Design review of the part built by this model. Coordinates are the model's own, in mm. A direction names the side the tool comes from. Give positions to 0.01 mm unless a question says otherwise; leave off trailing zeros. Loops run counter-clockwise (first coordinate to the right, second up) from the corner with the lowest first, then second, coordinate; pieces in that order, holes last.
Autodesk Inventor part; units mm, degrees
ref_plane "YZ Plane" through (0, 0, 0) normal (1, 0, 0) x (0, 1, 0)
ref_plane "XZ Plane" through (0, 0, 0) normal (0, 1, 0) x (-1, 0, 0)
ref_plane "XY Plane" through (0, 0, 0) normal (0, 0, 1) x (1, 0, 0)
sketch "スケッチ2" plane through (0, 0, 0) normal (0, 1, 0) x (-1, 0, 0)
  line L0 (-32.5, -11.25) -> (32.5, -11.25)
  line L1 (32.5, -11.25) -> (32.5, 11.25)
  line L2 (32.5, 11.25) -> (-32.5, 11.25)
  line L3 (-32.5, 11.25) -> (-32.5, -11.25)
  line L4 (-32.5, -11.25) -> (32.5, 11.25) construction
  line L5 (32.5, -11.25) -> (-32.5, 11.25) construction
  line L6 (-30, -8.75) -> (30, -8.75)
  line L7 (30, -8.75) -> (30, 8.75)
  line L8 (30, 8.75) -> (-30, 8.75)
  line L9 (-30, 8.75) -> (-30, -8.75)
  line L10 (-30, -8.75) -> (30, 8.75) construction
  line L11 (30, -8.75) -> (-30, 8.75) construction
  circle A0 centre (30, 8.75) radius 2.5
  circle A1 centre (30, -8.75) radius 2.5
  circle A2 centre (-30, 8.75) radius 2.5
  circle A3 centre (-30, -8.75) radius 2.5
  line L12 (-115, -18.25) -> (115, -18.25)
  line L13 (115, -18.25) -> (115, 18.25)
  line L14 (115, 18.25) -> (-115, 18.25)
  line L15 (-115, 18.25) -> (-115, -18.25)
  line L16 (-115, -18.25) -> (115, 18.25) construction
  line L17 (115, -18.25) -> (-115, 18.25) construction
  line L18 (-95, -18.25) -> (95, -18.25)
  line L19 (95, -18.25) -> (95, 18.25)
  line L20 (95, 18.25) -> (-95, 18.25)
  line L21 (-95, 18.25) -> (-95, -18.25)
  line L22 (-95, -18.25) -> (95, 18.25) construction
  line L23 (95, -18.25) -> (-95, 18.25) construction
  point P0 (0, 0)
  dimension "d10" = 65
  dimension "d11" = 22.5
  dimension "d12" = 60
  dimension "d13" = 17.5
  dimension "d14" = 230
  dimension "d15" = 36.5
  dimension "d16" = 190
sketch "スケッチ4" plane through (0, 0, 0) normal (1, 0, 0) x (0, 1, 0)
  point P0 (0, 0)
sketch "スケッチ5" plane through (0, 0, 0) normal (1, 0, 0) x (0, 1, 0)
  circle A0 centre (0, 0) radius 18.25
  line L0 (0, 0) -> (0, 6)
  line L1 (0, 6) -> (0, -6)
  circle A1 centre (0, 6) radius 3
  circle A2 centre (0, -6) radius 9
  circle A3 centre (0, 6) radius 9
  circle A4 centre (0, -6) radius 3
  line L2 (0, 6) -> (5.2915, 0)
  circle A5 centre (5.2915, 0) radius 5
  circle A6 centre (5.2915, 0) radius 4.5
  circle A7 centre (5.2915, 0) radius 5.5
  line L3 (0, 0) -> (0, 11.25)
  line L4 (0, 11.25) -> (0, -11.25)
  line L5 (5.2915, 5.5) -> (5.2915, -5.5)
  line L6 (0, 11.25) -> (-1.2, 11.25)
  line L7 (-1.2, 11.25) -> (-1.2, -11.25)
  line L8 (-1.2, -11.25) -> (0, -11.25)
  line L9 (-1.2, 11.25) -> (-9.2, 11.25)
  line L10 (-1.2, -11.25) -> (-9.2, -11.25)
  line L11 (-9.2, -11.25) -> (-9.2, 11.25)
  line L12 (-9.2, 11.25) -> (-10.4, 11.25)
  line L13 (-10.4, 11.25) -> (-10.4, -11.25)
  line L14 (-10.4, -11.25) -> (-9.2, -11.25)
  circle A8 centre (0, 0) radius 16
  line L15 (0, 11.25) -> (1.5, 11.25)
  line L16 (1.5, 11.25) -> (1.5, -11.25)
  line L17 (1.5, -11.25) -> (0, -11.25)
  line L18 (5.2915, 5.5) -> (1.5, 5.5)
  line L19 (5.2915, -5.5) -> (1.5, -5.5)
  circle A9 centre (5.2915, 0) radius 6.6802
  point P0 (0, 1.5)
  point P1 (0, -1.5)
  point P2 (1.5, -3.9843)
  point P3 (1.5, 3.9843)
  dimension "d28" = 36.5
  dimension "d29" = 6
  dimension "d30" = 12
  dimension "d31" = 6
  dimension "d32" = 18
  dimension "d33" = 8
  dimension "d34" = 9
  dimension "d35" = 11
  dimension "d36" = 11.25
  dimension "d37" = 22.5
  dimension "d39" = 1.2
  dimension "d40" = 8
  dimension "d41" = 1.2
  dimension "d42" = 32
  dimension "d43" = 1.5
extrude "押し出し1" add sketch "スケッチ5" against normal blind 5 contours L0 A7 A2 A5 A3 L1 | L0 A2 A7 | A7 A3 L1 | L0 A9 L2 L16 A7 A1 | A1 A7 A2 | A7 A1 L16 A5 A2 | A4 A7 L16 A9 L1 | A3 A7 A4 | A3 A5 L16 A4 A7 | L0 L2 A9 | A7 L16 A1 | A5 L16 A2 | A2 L16 A6 A3 A5 | A9 L16 A4 L4 L1 | A4 L16 A7 | A3 L16 A5 | L3 A1 L16 A9 L2 | A9 L16 L2 | L3 L15 L16 A1 | L16 A6 | A4 L16 L17 L4 picked at (1.4091, -3.6973)
extrude "押し出し2" add sketch "スケッチ5" against normal blind 3 contours L0 A7 A2 A5 A3 L1 | A7 A1 L16 A5 A2 | A3 A5 L16 A4 A7 | A7 L16 A1 | A5 L16 A2 | A2 L16 A6 A3 A5 | A4 L16 A7 | A3 L16 A5 | L16 A7 L2 A1 | A1 A5 L16 | L16 L2 A7 | L16 A5 L2 A6 A2 | A2 A6 L16 | L16 A7 A4 L19 | L16 A5 A4 | A4 A7 L16 | L16 A6 A3 | A3 A6 L5 A5 L16 | L16 L18 A1 A7 L2 | L2 A7 A1 | A5 L5 A6 L2 | A1 A7 L5 A5 | A6 L2 A2 | A2 L2 L5 A3 A6 L16 | L16 A6 | A4 A7 L19 | A5 L5 A7 A4 | A3 L5 A6 | L18 A7 A1 | A6 L5 A2 L2 | L5 A7 A3 A5 | A5 A3 A6 L5 | A2 L5 L2 | L5 A5 A2 A7 | L5 A6 A2 A5 | L5 A2 A3 | A3 A2 A6 L5 | A6 A3 A2 L5 | A5 A2 A6 A3 | A3 A7 A2 A5 | A3 A6 A2
extrude "押し出し3" add sketch "スケッチ5" along normal blind 16.5 contours L1 A7 L0 | L0 A7 A2 A5 A3 L1 | A7 L1 A3 A9 L7 A2 L0 | L0 A2 A7 | A7 A3 L1 | A1 A9 L0 | A2 A9 A1 | L0 A9 L2 L16 A7 A1 | A1 A7 A2 | A7 A1 L16 A5 A2 | A4 A7 L16 A9 L1 | A4 A9 A3 | A3 A7 A4 | L1 A9 A4 | A3 A5 L16 A4 A7 | A7 L16 A1 | A5 L16 A2 | A2 L16 A6 A3 A5 | A4 L16 A7 | A3 L16 A5 | A9 L16 L2 | L16 A7 L2 A1 | A1 A5 L16 | L16 L2 A7 | L7 A9 | L16 A5 L2 A6 A2 | A2 A6 L16 | L16 A7 A4 L19 | L16 A5 A4 | A4 A7 L16 | L16 A6 A3 | A3 A6 L5 A5 L16 | L16 L18 A1 A7 L2 | L2 A7 A1 | A5 L5 A6 L2 | A1 A7 L5 A5 | A6 L2 A2 | A2 L2 L5 A3 A6 L16 | L16 A6 | A4 A7 L19 | A5 L5 A7 A4 | A3 L5 A6 | L18 A7 A1 | A6 L5 A2 L2 | L5 A7 A3 A5 | A5 A3 A6 L5 | A2 L5 L2 | L5 A5 A2 A7 | L5 A6 A2 A5 | L5 A2 A3 | A3 A2 A6 L5 | A6 A3 A2 L5 | A5 A2 A6 A3 | A3 A7 A2 A5 | A3 A6 A2
extrude "押し出し4" cut sketch "スケッチ5" along normal blind 16.5 contours A6 L2 A2 | A2 L2 L5 A3 A6 L16 | L16 A6 | A3 L5 A6 | A6 L5 A2 L2 | A2 L5 L2 | L5 A2 A3 | A3 A2 A6 L5 | A6 A3 A2 L5 | A3 A6 A2
extrude "押し出し5" cut sketch "スケッチ5" against normal blind 1.5 contours A6 L2 A2 | A2 L2 L5 A3 A6 L16 | L16 A6 | A3 L5 A6 | A6 L5 A2 L2 | A2 L5 L2 | L5 A2 A3 | A3 A2 A6 L5 | A6 A3 A2 L5 | A3 A6 A2
sketch "スケッチ6" plane through (16.5, 5.2915, 0) normal (1, 0, 0) x (0, 0, 1)
  line L0 (0, 5.2915) -> (6, 5.2915)
  line L1 (-11.25, 5.2915) -> (11.25, 5.2915)
  line L2 (6, 5.2915) -> (-6, 5.2915)
  circle A0 centre (6, 5.2915) radius 1.05
  circle A1 centre (-6, 5.2915) radius 1.05
  circle A2 centre (0, 5.2915) radius 16
  circle A3 centre (0, 0) radius 5
  line L3 (0, 0) -> (0, 3)
  line L4 (0, 3) -> (0, -5.5)
  arc A4 (-5.5, 0) -> (5.5, 0) centre (0, 0) ccw
  line L5 (0, 3) -> (1, 3)
  line L6 (1, 3) -> (-1, 3)
  line L7 (-1, 3) -> (-1, -5.4083)
  line L8 (1, 3) -> (1, -5.4083)
  circle A5 centre (6, 5.2915) radius 9
  circle A6 centre (-6, 5.2915) radius 9
  line L9 (0, 5.2915) -> (0, -2.7085)
  circle A7 centre (0, -2.7085) radius 8
  circle A8 centre (6, 5.2915) radius 10
  circle A9 centre (-6, 5.2915) radius 10
  line L10 (0, 5.2915) -> (0, -5.7085)
  line L11 (0, -5.7085) -> (-11.619, -5.7085)
  line L12 (0, -5.7085) -> (11.619, -5.7085)
  line L13 (0, -5.7085) -> (9.5, -5.7085)
  line L14 (9.5, -5.7085) -> (-9.5, -5.7085)
  circle A10 centre (0, 5.2915) radius 18
  line L15 (1, -5.4083) -> (1, -8.2085)
  line L16 (-1, -5.4083) -> (-1, -8.2085)
  line L17 (0, 5.2915) -> (0, 6.4915)
  line L18 (0, 6.4915) -> (0, 14.4915)
  line L19 (0, 14.4915) -> (0, 15.6915)
  line L20 (0, 15.6915) -> (-11.25, 15.6915)
  line L21 (-11.25, 15.6915) -> (11.25, 15.6915)
  line L22 (11.25, 15.6915) -> (11.25, 14.4915)
  line L23 (11.25, 14.4915) -> (0, 14.4915)
  line L24 (-11.25, 14.4915) -> (-11.25, 15.6915)
  line L25 (0, 14.4915) -> (-11.25, 14.4915)
  line L26 (0, 15.6915) -> (8.75, 15.6915)
  line L27 (8.75, 15.6915) -> (-8.75, 15.6915)
  line L28 (11.25, 15.6915) -> (11.25, 17.1915)
  line L29 (11.25, 17.1915) -> (-11.25, 17.1915)
  line L30 (-11.25, 17.1915) -> (-11.25, 15.6915)
  line L31 (6, 17.1915) -> (6, 18.6915)
  line L32 (-6, 17.1915) -> (-6, 18.6915)
  circle A11 centre (6, 18.6915) radius 2.5
  circle A12 centre (-6, 18.6915) radius 2.5
  line L33 (6, 21.1915) -> (-6, 21.1915)
  line L34 (9.5, -5.7085) -> (12, -5.7085)
  line L35 (-9.5, -5.7085) -> (-12, -5.7085)
  line L36 (6, 18.6915) -> (8.5, 18.6915)
  line L37 (-6, 18.6915) -> (-8.5, 18.6915)
  circle A13 centre (0, 0) radius 4.5
  circle A14 centre (-6, 5.2915) radius 1.5
  circle A15 centre (6, 5.2915) radius 1.5
  circle A16 centre (6, 18.6915) radius 1.65
  circle A17 centre (-6, 18.6915) radius 1.65
  line L38 (9.5, -5.7085) -> (9.5, -6.2085)
  line L39 (9.5, -6.2085) -> (-9.5, -6.2085)
  line L40 (-9.5, -6.2085) -> (-9.5, -5.7085)
  circle A18 centre (-9.5, -6.2085) radius 1.65
  circle A19 centre (9.5, -6.2085) radius 1.65
  circle A20 centre (9.5, -6.2085) radius 2.5
  circle A21 centre (-9.5, -6.2085) radius 2.5
  line L41 (-12, -6.2085) -> (-8.5, 18.6915)
  line L42 (12, -6.2085) -> (8.5, 18.6915)
  line L43 (9.5, -8.7085) -> (-9.5, -8.7085)
  line L44 (1, -8.7085) -> (1, -8.0358)
  line L45 (-1, -8.7085) -> (-1, -8.2085)
  point P0 (1, -4.3875)
  point P1 (-1, -4.3875)
  point P2 (-4.4567, 20.6583)
  point P3 (-8.495, 18.8501)
  point P4 (4.4567, 20.6583)
  point P5 (8.495, 18.8501)
  point P6 (1.7861, 21.1915)
  point P7 (-1.7861, 21.1915)
  point P8 (11.9031, -5.5193)
  point P9 (11.8759, -5.4306)
  point P10 (11.8887, -5.4164)
  dimension "d54" = 6
  dimension "d55" = 12
  dimension "d56" = 2.1
  dimension "d57" = 2.1
  dimension "d58" = 32
  dimension "d59" = 10
  dimension "d60" = 3
  dimension "d61" = 1
  dimension "d62" = 2
  dimension "d65" = 18
  dimension "d66" = 18
  dimension "d67" = 8
  dimension "d68" = 11
  dimension "d69" = 9.5
  dimension "d70" = 19
  dimension "d73" = 36
  dimension "d76" = 1.2
  dimension "d77" = 8
  dimension "d78" = 1.2
  dimension "d79" = 8.75
  dimension "d80" = 17.5
  dimension "d81" = 1.5
  dimension "d82" = 1.5
  dimension "d83" = 5
  dimension "d84" = 5
  dimension "d97" = 3
  dimension "d98" = 3
  dimension "d109" = 3.3
  dimension "d110" = 3.3
  dimension "d111" = 0.5
  dimension "d112" = 3.3
  dimension "d113" = 3.3
  dimension "d114" = 5
  dimension "d115" = 5
extrude "押し出し6" cut sketch "スケッチ6" against normal blind 19.5 contours L5 L8 A6 L4 L3 | L3 L4 A5 L7 L6 | L8 A9 A5 A6 | A5 A6 A8 L7 | L8 A5 A9 | A5 A9 L4 | L4 A8 A6 | A8 A6 L7 | L8 A8 A9 A5 | A8 L8 A13 L4 | A9 L7 A6 A8 | L4 A13 L7 A9 | L7 A13 L4 A3 | A3 L4 A4 L7 | L8 A4 L4 A3 | A3 L4 A13 L8
sketch "スケッチ7" plane through (-5, 1.5, -11.25) normal (0, 1, 0) x (1, 0, 0)
  line L0 (0, 0) -> (2.5, 0)
  line L1 (5, 0) -> (0, 0)
  line L2 (2.5, 0) -> (2.5, -22.5)
  line L3 (5, -22.5) -> (0, -22.5)
  line L4 (2.5, 0) -> (2.5, -2.5)
  line L5 (2.5, -2.5) -> (2.5, -20)
  point P0 (5, -11.25)
  dimension "d87" = 2.5
  dimension "d88" = 17.5
hole "穴1" at (-2.5, 1.5, -8.75) at (-2.5, 1.5, 8.75) direction (0, -1, 0) diameter 2 end through all
fillet "フィレット1" radius 2 2 edges at (0, 0.75, -11.25) (0, 0.75, 11.25)
extrude "押し出し11" add sketch "スケッチ6" against normal blind 4 contours L17 L18 A6 L0 | A7 A5 L1 | A7 A6 A3 L9 | L0 A6 A7 | L9 A3 A5 A7 | L1 A5 L18 L17 | A6 A5 A9 L0 | L0 A9 A7 A6 | A5 A7 A8 L1 | L1 A8 A6 A5 | L9 A13 A5 A3 | A3 A6 A13 L9 | A7 A9 A3 A6 | A5 A3 A8 A7 | A9 A5 L42 L1 A15 L0 | L0 A15 L1 L42 A5 A7 A9 | L18 A9 A5 | A6 A8 L18 | A8 A7 A6 L41 L1 A14 | L1 A14 L41 A6 A8 | A3 A9 A13 A6 | A5 A13 A8 A3 | A7 A5 A3 A9 | A8 A3 A6 A7 | A15 L1 A0 L0 | L0 A0 L1 A15 | A9 A8 L23 L42 A5 | A6 L41 L25 A9 A8 | L18 L23 A8 | A9 L25 L18 | A14 L1 A1 | L1 A1 A14 | A3 A5 A13 A9 | A8 A13 A6 A3 | A7 A21 A9 L41 A6 | A6 A4 A9 A21 A7 | L23 L19 L21 L42 A8 | A8 L42 L23 | L25 L41 A9 | A9 L41 L20 L19 L25 | A6 A13 A9 A3 | A3 A9 A4 A6 | A7 A20 A8 A4 A5 | A5 L42 A8 A20 A7 | A21 A9 A7 | A7 A9 A21 | L20 L41 L29 A12 A11 L42 L21 | A5 A4 A8 A3 | A3 A8 A13 A5 | A9 A13 L7 A3 | A3 L7 A4 A9 | A20 A8 A7 | A7 A8 A20 | A9 A21 A2 L41 | A4 L16 L11 A21 A9 | A9 A21 L11 A7 | A7 L11 A18 A2 A21 A9 | A8 A4 L8 A3 | A3 L8 A13 A8 | A8 A20 L12 L15 A4 | L42 A2 A20 A8 | A8 A20 A2 L12 A19 A7 | A7 L12 A20 A8 | A2 A21 L41 | L11 A21 L39 A7 | A7 L39 A18 L11 | L11 L16 L39 A21 | A2 L35 L41 A21 | L29 A11 L42 | L41 A12 L29 | L12 A19 L39 A7 | A7 L39 A20 L12 | A20 L42 L34 A2 | A20 L39 L15 L12 | L39 A21 A7 | A7 A21 A2 A18 L39 | L39 L16 L45 L43 A7 A21 | L11 A18 A2 | A2 A18 A21 L41 L35 | A11 L29 A16 | L29 A16 L36 A11 | L36 A16 A2 A11 | A12 L37 A17 L29 | L29 A17 A12 | A12 A2 A17 L37 | L39 A19 A2 A20 A7 | A7 A20 L39 | L34 L42 A20 A2 A19 | A2 A19 L12 | A20 A7 L43 L44 L15 L39 | A7 L43 A2 A21 | A2 A16 A11 | A11 A2 A16 L29 | L29 A12 A2 L33 A11 | L29 A17 A2 A12 | A12 A2 A17 | A20 A2 L43 A7 | A2 L43 A21 | A11 A2 L33 | L33 A2 A12 | A20 L43 A2 picked at (5.1751, 14.7127) picked at (-5.1751, 14.7127)
properties part number "ikafly1a"
Q1. Tool access review of faces 1 (the face through (4.64, 8.77, 4.26)), 2 (the face through (-0.6, 0.74, -10.68)), 3 (the face through (7, 10, -1)): name each direction out of +Z, -Z, +X, -X, +Y, -Y from which nothing blocks a thin tool from reaching the whole face with its end or side.
Results:
face 1: +Z, -X, +Y
face 2: -Z, +Y, -Y
face 3: +X, -X, +Y
Q2. Insertion check: pin 1 (1.9 mm diameter, centred on y = 0, z = -6, fed in from +X); pin 2 (4 mm diameter, centred on y = -13.4, z = -6, fed in from +X); pin 3 (3 mm diameter, centred on x = -2.5, z = -8.75, fed in from -Y); pin 4 (10 mm diameter, centred on x = 5.5, y = -1.5, fed in from +Z). Each pin has a flat end and moves straight along its axis. Give the tip position at first contact, or say it passes through.
Results:
pin 1: stops at x = 0
pin 2: stops at x = 16.5
pin 3: stops at y = 0
pin 4: stops at z = 5.5
Q3. Take a section at B-B (y = 4.25). Give the boundary of the cut face in (x, z).
Results:
outline: (-3, -5.5) - (12.5, -5.5) - (12.5, -10.98) - (16.5, -10.98) - (16.5, -4.38) - (-1.5, -4.38) - (-1.5, -1) - (-3, -1) - close; (-3, 1) - (-1.5, 1) - (-1.5, 4.38) - (16.5, 4.38) - (16.5, 10.98) - (12.5, 10.98) - (12.5, 5.5) - (-3, 5.5) - close
Q4. Draft analysis for pull direction Z (two halves, no side actions). For faces 4 (the face through (6.16, -1.39, -0.09)), 5 (the face through (7.374, 0.795, -0.184)), 6 (the face through (14.528, -15.187, -7.748)), 7 (the face through (-2, 2.292, 0)), state which applies: pulls with the +Z half, pulls with the -Z half, needs draft (parallel to the pull), parting line crosses it, or undercut.
Results:
face 4: parting line crosses it
face 5: undercut
face 6: pulls with the -Z half
face 7: undercut
Q5. Take a section at C-C (x = 3.25). Give the boundary of the cut face in (y, z).
Results:
outline: (1.5, -5.5) - (5.29, -5.5) arc R5.5 ccw to (10.7, -1) - (9.68, -1) arc R4.5 cw (long way) to (9.68, 1) - (10.7, 1) arc R5.5 ccw to (5.29, 5.5) - (1.5, 5.5) arc R6.68 ccw to start
Q6. Take a section at A-A (x = 14.5). Give the number of separate pieces and of enclosed holes in the cut face, plus the area to 3 significant figures.
Results:
separate pieces: 1
enclosed holes: 6
area: 494 mm2
Q7. Take a section at D-D (y = -9). Give the boundary of the cut face in (x, z), plus the area to 3 significant figures.
Results:
outline: (12.5, -9.12) - (16.5, -9.12) - (16.5, 9.12) - (12.5, 9.12) - close
area: 72.9 mm2
Q8. Wall thickness on line 1 (Y direction, x = 14.4, z = -6); line 2 (Z direction, x = 14.95, y = 11.5); line 3 (Z direction, x = 15.1, y = -13.4): over which ranges is each line inside the solid? List them lowest first.
Results:
line 1: y = -15.9 to -15.05, -11.75 to -1.05, 1.05 to 14
line 2: z = -12 to -11.15, -7.85 to -1, 1 to 7.85, 11.15 to 12
line 3: z = -8.5 to -7.65, -4.35 to 4.35, 7.65 to 8.5
